The listing builds one solid part. Answer for the finished solid, in the listing's coordinates (mm). Give positions to 0.01 mm unless a question says otherwise; leave off trailing zeros. Write each loop counter-clockwise with the first axis right and the second up, starting at its lowest first coordinate (ties: lowest second). Pieces come first, ordered by that corner, then holes.
```python
from build123d import *

# Parameters (mm, degrees)
BOSS_EXTRUDE1_DEPTH   = 3
BODY_MOVE_COPY1_ANGLE = 90
CUT_EXTRUDE2_REACH    = 84.517
SKETCH8_R             = 1.05
SKETCH8_R_2           = 0.75


with BuildPart() as part:
    # Sketch1 → Boss-Extrude1 (new body)
    with BuildSketch(Plane(origin=(0, 0, 0), x_dir=(1, 0, 0), z_dir=(0, 1, 0))):
        with BuildLine():
            Line((50, -20), (0, -20))
            ThreePointArc((0, -20), (-20, 0), (0, 20))
            Line((0, 20), (50, 20))
            Line((50, 20), (80, 0.010830805))
            Line((80, 0.010830805), (80, 0))
            Line((80, 0), (50, -20))
        make_face()
    extrude(amount=BOSS_EXTRUDE1_DEPTH)


with BuildPart() as part_1:
    # Body-Move/Copy1: moved
    add(part.part.rotate(Axis((0, 0, 0), (1, 0, 0)), BODY_MOVE_COPY1_ANGLE))

    # Sketch8 → Cut-Extrude2 (cut, up to next)
    with BuildSketch(Plane.XY.offset(3), mode=Mode.PRIVATE) as cut_extrude2_sk1:
        Circle(SKETCH8_R)
    cut_extrude2_tool1 = extrude(cut_extrude2_sk1.sketch, amount=-CUT_EXTRUDE2_REACH, mode=Mode.PRIVATE) & part_1.part
    # Sketch8 → Cut-Extrude2 (cut, up to next)
    with BuildSketch(Plane.XY.offset(3), mode=Mode.PRIVATE) as cut_extrude2_sk2:
        with Locations((6, -0.032589943)):
            Circle(SKETCH8_R_2)
    cut_extrude2_tool2 = extrude(cut_extrude2_sk2.sketch, amount=-CUT_EXTRUDE2_REACH, mode=Mode.PRIVATE) & part_1.part
    # Sketch8 → Cut-Extrude2 (cut, up to next)
    with BuildSketch(Plane.XY.offset(3), mode=Mode.PRIVATE) as cut_extrude2_sk3:
        with Locations((-5.999934973, 0.027934237)):
            Circle(SKETCH8_R_2)
    cut_extrude2_tool3 = extrude(cut_extrude2_sk3.sketch, amount=-CUT_EXTRUDE2_REACH, mode=Mode.PRIVATE) & part_1.part
    add(cut_extrude2_tool1.solids().sort_by_distance((0, 0, 3))[0], mode=Mode.SUBTRACT)
    add(cut_extrude2_tool2.solids().sort_by_distance((6, -0.03259, 3))[0], mode=Mode.SUBTRACT)
    add(cut_extrude2_tool3.solids().sort_by_distance((-5.999935, 0.027934, 3))[0], mode=Mode.SUBTRACT)


with BuildPart() as part_2:
    # Body-Move/Copy4: moved
    add(part_1.part.moved(Location((0, 0, -3))))


solid = part_2.part
```
Item 1: Determine the mould class of faces 1 (the face through (-20, 0, -2)), 2 (the face through (1, 0.32, -1.48)), 3 (the face through (25, 20, -2)) for opening direction X: pulls with the +X half, pulls with the -X half, needs draft (parallel to the pull), parting line crosses it, or undercut.
Conclusion:
face 1: pulls with the -X half
face 2: undercut
face 3: needs draft
Item 2: A cutting plane is placed at A-A, the plane z = -0.7. Count the separate pieces of the cut face and the enclosed holes in it, plus the area to 3 significant figures.
Conclusion:
separate pieces: 1
enclosed holes: 3
area: 3,220 mm2
Item 3: This flat-tipped pin is pushed along its axis until it touches: P1, Ø1.2, axis at x = 6, y = -0.03, coming from the +Z side. Where does it stop, or does it pass through?
Conclusion:
P1: passes through
Item 4: A cutting plane is placed at C-C, the plane y = 9. Give the vertices of the cut face in (x, z).
Conclusion:
outline: (-17.86, -3) - (66.51, -3) - (66.51, 0) - (-17.86, 0) - close
Item 5: Consider probe 1 along Y at (x, z) = (6, -1.6); probe 2 along Y at (x, z) = (0, -1.4); probe 3 along X at (y, z) = (-11.5, -2.05). Determine where each line is inside the solid, lowest interval first.
Conclusion:
probe 1: y = -20 to -0.78, 0.72 to 20
probe 2: y = -20 to -1.05, 1.05 to 20
probe 3: x = -16.36 to 62.75
Item 6: A cutting plane is placed at B-B, the plane y = -2.5. Give the vertices of the cut face in (x, z), plus the area to 3 significant figures.
Conclusion:
outline: (-19.84, -3) - (76.25, -3) - (76.25, 0) - (-19.84, 0) - close
area: 288 mm2
